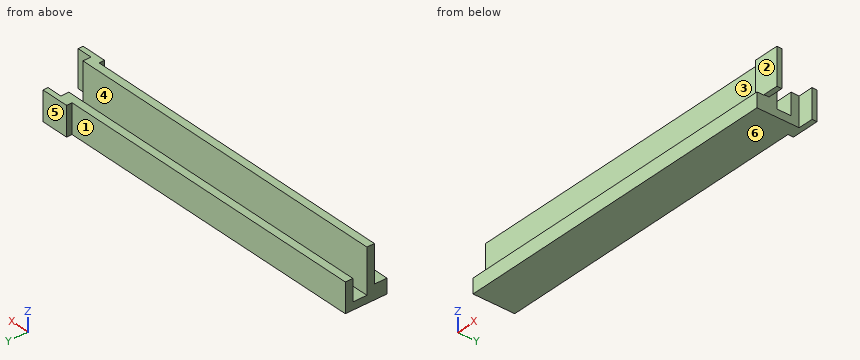
from build123d import *

# Parameters (mm, degrees)
F0_W      = 133
F0_H      = 11.6
F1_DEPTH  = 11.6
F2_W      = 5.6
F2_H      = 8.6
F3_DEPTH  = 133
F4_DEPTH  = 9
F5_W      = 133
F5_H      = 5.8
F6_DEPTH  = 5
F8_W      = 4
F8_H      = 14.8
F9_DEPTH  = 2.2
F10_W     = 2
F10_H     = 14.6
F11_DEPTH = 6
F12_W     = 5
F12_H     = 11.6
F13_DEPTH = 2.2
F14_W     = 2
F14_H     = 11.6
F15_DEPTH = 6


with BuildPart() as f1:
    # F0 (on Front) → F1 (new body)
    with BuildSketch(Plane.XZ):
        Rectangle(F0_W, F0_H)
    extrude(amount=F1_DEPTH)

    # F2 (on face) → F3 (cut)
    with BuildSketch(Plane.YZ.offset(66.5)):
        with Locations((-5.8, 1.5)):
            Rectangle(F2_W, F2_H)
    extrude(amount=-F3_DEPTH, mode=Mode.SUBTRACT)

    # F4 (add): a face of the model
    f4_faces = [f1.faces().sort_by_distance(p)[0] for p in [
        (0, -10.1, 5.8),
    ]]
    extrude(f4_faces, amount=F4_DEPTH)

    # F5 (on face) → F6 (join)
    with BuildSketch(Plane.XZ.offset(11.6)):
        with Locations((0, -2.9)):
            Rectangle(F5_W, F5_H)
    extrude(amount=F6_DEPTH)

    # F8 (on face) → F9 (join)
    with BuildSketch(Plane.XZ.offset(11.6)):
        with Locations((64.5, 7.4)):
            Rectangle(F8_W, F8_H)
    extrude(amount=F9_DEPTH)

    # F10 (on face) → F11 (join)
    with BuildSketch(Plane.YZ.offset(66.5)):
        with Locations((-12.8, 7.5)):
            Rectangle(F10_W, F10_H)
    extrude(amount=F11_DEPTH)

    # F12 (on face) → F13 (join)
    with BuildSketch(Plane(origin=(0, 0, 0), x_dir=(-1, 0, 0), z_dir=(0, 1, 0))):
        with Locations((-64, 0)):
            Rectangle(F12_W, F12_H)
    extrude(amount=F13_DEPTH)

    # F14 (on face) → F15 (join)
    with BuildSketch(Plane.YZ.offset(66.5)):
        with Locations((1.2, 0)):
            Rectangle(F14_W, F14_H)
    extrude(amount=F15_DEPTH)


solid = f1.part
Build history of the part. All positions in model axes, mm. Face numbers are marked on the shaded views. A direction names the side the tool comes from. Round coordinates to 2 decimals unless told otherwise and drop trailing zeros. Write each loop counter-clockwise with the first axis right and the second up, starting at its lowest first coordinate (ties: lowest second). Pieces come first, ordered by that corner, then holes. Notation, with made-up numbers: M -34.5,44.5 L 3.5,44.5 A28 cw 3.5,81.5 Z; hole C 28.25,89.5 d10. An arc over 180 degrees is marked long. Use CSV: the item, a comma, the result in double quotes.
1. Saw through at C-C (z = 8.5). Give the cut face in (x, y), plus the area to 3 significant figures.
Reply:
outline,"M -66.5,-11.6 L 62.5,-11.6 L 62.5,-13.8 L 72.5,-13.8 L 72.5,-11.8 L 66.5,-11.8 L 66.5,-8.6 L -66.5,-8.6 Z"
area,"420 mm²"
2. Flat gauge pins, fed straight in: pin 1 (2.5 mm diameter, centred on y = 1.5, z = -1.5, fed in from -X); pin 2 (5.5 mm diameter, centred on x = 4.5, y = -15, fed in from +Z); pin 3 (9 mm diameter, centred on x = 24.5, z = 10, fed in from +Y). Where does each tip first touch, or does it go through?
Reply:
pin 1,"stops at x = 61.5"
pin 2,"stops at z = 0"
pin 3,"stops at y = 0"
3. Saw through at B-B (x = -52). Give the cut face in (y, z), plus the area to 3 significant figures.
Reply:
outline,"M -16.6,-5.8 L 0,-5.8 L 0,5.8 L -3,5.8 L -3,-2.8 L -8.6,-2.8 L -8.6,14.8 L -11.6,14.8 L -11.6,0 L -16.6,0 Z"
area,"142 mm²"
4. Saw through at A-A (z = 2.25). Give the cut face in (x, y).
Reply:
outline,"M -66.5,-11.6 L 62.5,-11.6 L 62.5,-13.8 L 72.5,-13.8 L 72.5,-11.8 L 66.5,-11.8 L 66.5,-8.6 L -66.5,-8.6 Z; M -66.5,-3 L 66.5,-3 L 66.5,0.2 L 72.5,0.2 L 72.5,2.2 L 61.5,2.2 L 61.5,0 L -66.5,0 Z"
5. Two-plate mould, pull along Y, no slides. Class the marked faces 3, 4, 5 and 6: +Y half, -Y half, draft (parallel to the pull), parting line (faces both ways), or undercut.
Reply:
face 3,"-Y half"
face 4,"undercut"
face 5,"+Y half"
face 6,"draft"
6. Tool access for the marked faces 1 and 2: list every direction of +Z, -Z, +X, -X, +Y, -Y with a clear straight run to the whole face (end or side of a thin tool).
Reply:
face 1,"+Z, -Z, -X, +Y"
face 2,"+Z, +X, -X, -Y"
7. Wall check: probe 1 along Y at (x, z) = (38, 0.5); probe 2 along Y at (x, z) = (-20, -0.75); probe 3 along X at (y, z) = (-12, 0.5). Give the ranges that are in metal, low to high. Write a range as from..to.
Reply:
probe 1,"y = -11.6..-8.6, -3..0"
probe 2,"y = -16.6..-8.6, -3..0"
probe 3,"x = 62.5..72.5"
